from build123d import *

# Parameters (mm, degrees)
BASPROSKE_W         = 3.175
BASPROSKE_H         = 5.291666667
TOOTHCUT_DEPTH      = 9.129212583
TEETHCUTS_COUNT     = 18
TEETHCUTS_ANGLE     = 340
SKETCH2_3_R         = 1.5875
BOSS_EXTRUDE1_DEPTH = 24.60625
SKETCH3_R           = 3.175
BOSS_EXTRUDE2_DEPTH = 1.5875


with BuildPart() as part:
    # BasProSke → Base-Revolve (revolve)
    with BuildSketch(Plane(origin=(0, 0, 0), x_dir=(1, 0, 0), z_dir=(0, 1, 0)), mode=Mode.PRIVATE) as base_revolve_sk:
        with Locations((1.5875, 2.645833334)):
            Rectangle(BASPROSKE_W, BASPROSKE_H)
    revolve(base_revolve_sk.sketch.rotate(Axis((-10, 0, 0), (1, 0, 0)), 180), axis=Axis((-10, 0, 0), (1, 0, 0)))

    # TooCutSke → ToothCut (cut, through all)
    with BuildSketch(Plane(origin=(0, 0, 0), x_dir=(0, 0, -1), z_dir=(1, 0, 0))):
        with BuildLine():
            ThreePointArc((0.270003318, 4.067748898), (0, 4.0767), (-0.270003318, 4.067748898))
            ThreePointArc((-0.270003318, 4.067748898), (-0.437425956, 4.709129954), (-0.814487039, 5.254313352))
            ThreePointArc((-0.814487039, 5.254313352), (0, 5.317066667), (0.814487039, 5.254313352))
            ThreePointArc((0.814487039, 5.254313352), (0.437425956, 4.709129954), (0.270003318, 4.067748898))
        make_face()
    toothcut = extrude(amount=TOOTHCUT_DEPTH, mode=Mode.SUBTRACT)

    # TeethCuts: ToothCut ×18 about axis
    teethcuts_axis = Axis((-10, 0, 0), (1, 0, 0))
    for i in range(1, TEETHCUTS_COUNT):
        add(toothcut.rotate(teethcuts_axis, i * TEETHCUTS_ANGLE / (TEETHCUTS_COUNT - 1)), mode=Mode.SUBTRACT)

    # Sketch2_3 → Boss-Extrude1 (add)
    with BuildSketch(Plane.ZY):
        with Locations(Location((0, 0, 0), (0, 0, 180))):
            Circle(SKETCH2_3_R)
    extrude(amount=BOSS_EXTRUDE1_DEPTH)

    # Sketch3 → Boss-Extrude2 (add)
    with BuildSketch(Plane.ZY):
        with Locations(Location((0, 0, 0), (0, 0, 180))):
            Circle(SKETCH3_R)
    extrude(amount=BOSS_EXTRUDE2_DEPTH)


solid = part.part
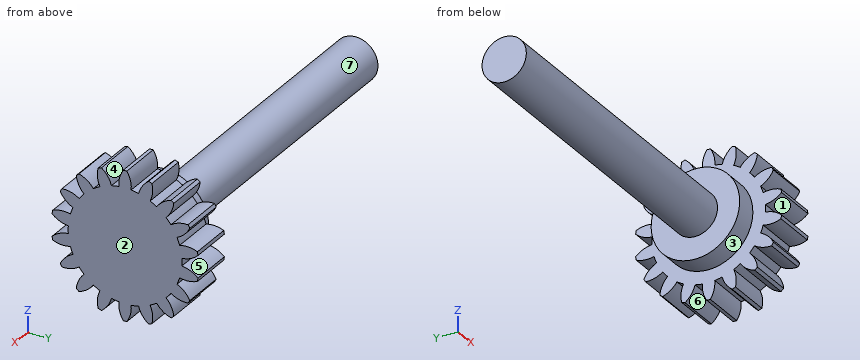
Geometry: final body of the model. Coordinates: model frame, mm. Face numbers are marked on the shaded views. A direction names the side the tool comes from. Round coordinates to 2 decimals unless told otherwise and drop trailing zeros. Loops run counter-clockwise (first coordinate to the right, second up) from the corner with the lowest first, then second, coordinate; pieces in that order, holes last.
Q1. Access query for the marked faces 4, 5, 6 and 7. Directions: +Z, -Z, +X, -X, +Y, -Y. A direction counts if a zero-diameter tool reaches every point of the face in a straight line with its end or side. Return the directions, or none.
Q2. Pull-direction query (Z, two-part tool) for the marked faces 1, 2 and 3; classes: released by +Z, released by -Z, zero draft, split by the parting line, or undercut.
Q3. Section B-B on x = -20.5. Return loops of the section in (y, z) (1 decimal), plus the area to 3 significant figures.
Q4. Section A-A on z = 0. Return loops of the section in (x, y) (1 decimal).
Q5. Pin query (flat end, axial travel): P1, Ø5, axis at y = -4, z = -3, coming from the -X side; P2, Ø5, axis at x = -3, z = -3.5, coming from the +Y side; P3, Ø1.5, axis at x = -1, z = 0, coming from the +Y side (3 decimals). Return the tip coordinate at first contact, or that it passes through.
Q6. Section C-C on x = -0.5. Return loops of the section in (y, z) (3 decimals), plus the area to 3 significant figures.
Q7. Material intervals for L1, parallel to X at y = 2.5, z = -1.25 (1 decimal); L2, parallel to Y at x = -5.75, z = 0; L3, parallel to X at y = 0.25, z = 4.75 (3 decimals), sorted ascending.
Evaluation:
1. face 4: +Z, +X, -X
1. face 5: +X, -X, +Y
1. face 6: -Z, +X, -X
1. face 7: -X
2. face 1: undercut
2. face 2: zero draft
2. face 3: split by the parting line
3. outline: circle Ø3.2 at (0, 0)
3. area: 7.92 mm2
4. outline: (-24.6, -1.6) - (-1.6, -1.6) - (-1.6, -3.2) - (0, -3.2) - (0, -4.1) - (3.2, -4.1) - (3.2, 4.1) - (0, 4.1) - (0, 3.2) - (-1.6, 3.2) - (-1.6, 1.6) - (-24.6, 1.6) - close
5. P1: stops at x = -1.59
5. P2: stops at y = 2.83
5. P3: stops at y = 3.175
6. outline: circle Ø6.35 at (0, 0)
6. area: 31.7 mm2
7. L1: x = -1.6 to 3.2
7. L2: y = -1.59 to 1.59
7. L3: x = 0 to 3.175
